```python
from build123d import *
from build123d.topology import SkipClean

# Parameters (mm, degrees)
SKETCH1_R           = 39.4
SKETCH1_R_2         = 30
BOSS_EXTRUDE1_DEPTH = 20
BOSS_EXTRUDE2_DEPTH = 15


with BuildPart() as part:
    # Sketch1 → Boss-Extrude1 (new body)
    with BuildSketch(Plane(origin=(0, 0, 0), x_dir=(1, 0, 0), z_dir=(0, 1, 0))):
        with Locations(Location((0, 0, 0), (0, 0, 270))):
            Circle(SKETCH1_R)
        with Locations(Location((0, 0, 0), (0, 0, 270))):
            Circle(SKETCH1_R_2, mode=Mode.SUBTRACT)
    extrude(amount=BOSS_EXTRUDE1_DEPTH)

    # Sketch2 → Boss-Extrude2 (add)
    with SkipClean():  # the faces are left unmerged after this step: merging them gives an invalid solid
        with BuildSketch(Plane(origin=(0, 20, 0), x_dir=(1, 0, 0), z_dir=(0, 1, 0))):
            with BuildLine():
                Line((-29.006131017, 7.657960788), (-38.094718735, 10.057455169))
                ThreePointArc((-38.094718735, 10.057455169), (-39.072317043, 5.070901391), (-39.4, 0))
                Line((-39.4, 0), (-30, 0))
                ThreePointArc((-30, 0), (-29.75049521, 3.861092429), (-29.006131017, 7.657960788))
            make_face()
            with BuildLine():
                Line((-27.21258864, -12.628341916), (-35.739199747, -16.585222382))
                ThreePointArc((-35.739199747, -16.585222382), (-32.295432702, -22.569116655), (-27.860007179, -27.860007179))
                Line((-27.860007179, -27.860007179), (-21.213203436, -21.213203436))
                ThreePointArc((-21.213203436, -21.213203436), (-24.590430992, -17.18460659), (-27.21258864, -12.628341916))
            make_face()
            with BuildLine():
                Line((-10.2606043, -28.190778624), (-13.475593647, -37.023889259))
                ThreePointArc((-13.475593647, -37.023889259), (-6.8417382, -38.801425469), (0, -39.4))
                Line((0, -39.4), (0, -30))
                ThreePointArc((0, -30), (-5.20944533, -29.54423259), (-10.2606043, -28.190778624))
            make_face()
            with BuildLine():
                Line((13.833981995, -26.619935052), (18.168629687, -34.960848034))
                ThreePointArc((18.168629687, -34.960848034), (23.286569909, -31.782002169), (27.860007179, -27.860007179))
                Line((27.860007179, -27.860007179), (21.213203436, -21.213203436))
                ThreePointArc((21.213203436, -21.213203436), (17.730890794, -24.199494037), (13.833981995, -26.619935052))
            make_face()
            with BuildLine():
                Line((39.4, 0), (30, 0))
                ThreePointArc((30, 0), (29.751894914, -3.850292074), (29.011683396, -7.636899012))
                Line((29.011683396, -7.636899012), (38.10201086, -10.029794035))
                ThreePointArc((38.10201086, -10.029794035), (39.07415532, -5.056716924), (39.4, 0))
            make_face()
            with BuildLine():
                Line((27.860007179, 27.860007179), (21.213203436, 21.213203436))
                ThreePointArc((21.213203436, 21.213203436), (24.686675185, 17.046057265), (27.352889551, 12.321502878))
                Line((27.352889551, 12.321502878), (35.923461611, 16.182240447))
                ThreePointArc((35.923461611, 16.182240447), (32.42183341, 22.387155208), (27.860007179, 27.860007179))
            make_face()
            with BuildLine():
                ThreePointArc((13.475593647, 37.023889259), (6.8417382, 38.801425469), (0, 39.4))
                Line((0, 39.4), (0, 30))
                ThreePointArc((0, 30), (5.20944533, 29.54423259), (10.2606043, 28.190778624))
                Line((10.2606043, 28.190778624), (13.475593647, 37.023889259))
            make_face()
            with BuildLine():
                ThreePointArc((-18.13649628, 34.977528539), (-23.271965112, 31.792697901), (-27.860007179, 27.860007179))
                Line((-27.860007179, 27.860007179), (-21.213203436, 21.213203436))
                ThreePointArc((-21.213203436, 21.213203436), (-17.71977039, 24.207637996), (-13.809514934, 26.632635943))
                Line((-13.809514934, 26.632635943), (-18.13649628, 34.977528539))
            make_face()
        extrude(amount=BOSS_EXTRUDE2_DEPTH)


solid = part.part
```
Could you check a few things on this model? Use its own coordinates, in mm. A direction names the side the tool comes from. Give positions to 0.01 mm unless a question says otherwise; leave off trailing zeros. Loops run counter-clockwise (first coordinate to the right, second up) from the corner with the lowest first, then second, coordinate; pieces in that order, holes last. Notation, with made-up numbers: (-12, -31) - (-6, -31) arc R20 ccw to (-6, -26) - close; hole circle Ø11 at (-32, -0.5). An arc over 180 degrees is marked (long way). Answer in a Markdown table with one row per item. Add a question column.
Q1. We'd pull the mould along Z, two halves only. Please class faces 4 (the face through (35, 27, 0)), 5 (the face through (0, 27, 35)), 6 (the face through (25, 27, -25)), 7 (the face through (31.578, 27.395, -14.225)): +Z half, -Z half, draft (parallel to the pull), parting line (faces both ways), or undercut.
Q2. If we section it at D-D (y = 10.5): List the corners of the cut face in (x, z) for me, plus the area to 3 significant figures.
Q3. If we section it at A-A (y = 28): State how many separate pieces and enclosed holes the cut face has, plus the area to 3 significant figures.
Q4. For pin 1 (3 mm diameter, centred on x = 33, y = 30, fed in from -Z); pin 2 (7.5 mm diameter, centred on y = 31, z = 35.5, fed in from +X); pin 3 (3 mm diameter, centred on x = -34, y = 25.5, fed in from +Z); pin 4 (5 mm diameter, centred on x = -22.5, z = -12, fed in from +Y), each with a flat end and sliding along its axis, tell me the tip position at first contact or that it passes through.
Q5. If we section it at C-C (x = -32): List the corners of the cut face in (y, z) for me, plus the area to 3 significant figures.
Q6. Which directions (+Z, -Z, +X, -X, +Y, -Y) give clear straight access to the entire face, cutting with the end or side of a thin tool? Please do faces 1 (the face through (33, 20, -8)), 2 (the face through (7, 20, 33)), 3 (the face through (11.846, 27.395, -32.546)).
Q7. If we section it at B-B (z = 9): List the corners of the cut face in (x, y) for me, plus the area to 3 significant figures.
Q8. Please list where these lines run through material, in increasing order: L1, parallel to X at y = 9.5, z = 0; L2, parallel to Y at x = 32.5, z = 14.5. Write a range as from..to.
The answers:
| question | item | result |
|---|---|---|
| 1 | face 4 | undercut |
| 1 | face 5 | draft |
| 1 | face 6 | -Z half |
| 1 | face 7 | undercut |
| 2 | outline | circle Ø78.8 at (0, 0); hole circle Ø60 at (0, 0) |
| 2 | area | 2,050 mm^2 |
| 3 | separate pieces | 8 |
| 3 | enclosed holes | 0 |
| 3 | area | 828 mm^2 |
| 4 | pin 1 | stops at z = -23.67 |
| 4 | pin 2 | stops at x = 23.33 |
| 4 | pin 3 | stops at z = 22.27 |
| 4 | pin 4 | passes through |
| 5 | outline | (0, -22.99) - (20, -22.99) - (20, -8.45) - (35, -8.45) - (35, 0) - (20, 0) - (20, 14.85) - (35, 14.85) - (35, 22.99) - (0, 22.99) - close |
| 5 | area | 1,170 mm^2 |
| 6 | face 1 | +X, +Y |
| 6 | face 2 | +Z, +Y |
| 6 | face 3 | +Z, +X, +Y |
| 7 | outline | (-38.36, 0) - (-28.62, 0) - (-28.62, 20) - (-38.36, 20) - close; (28.62, 0) - (38.36, 0) - (38.36, 35) - (34.19, 35) - (34.19, 20) - (28.62, 20) - close |
| 7 | area | 452 mm^2 |
| 8 | L1 | x = -39.4..-30, 30..39.4 |
| 8 | L2 | y = 0..20 |
